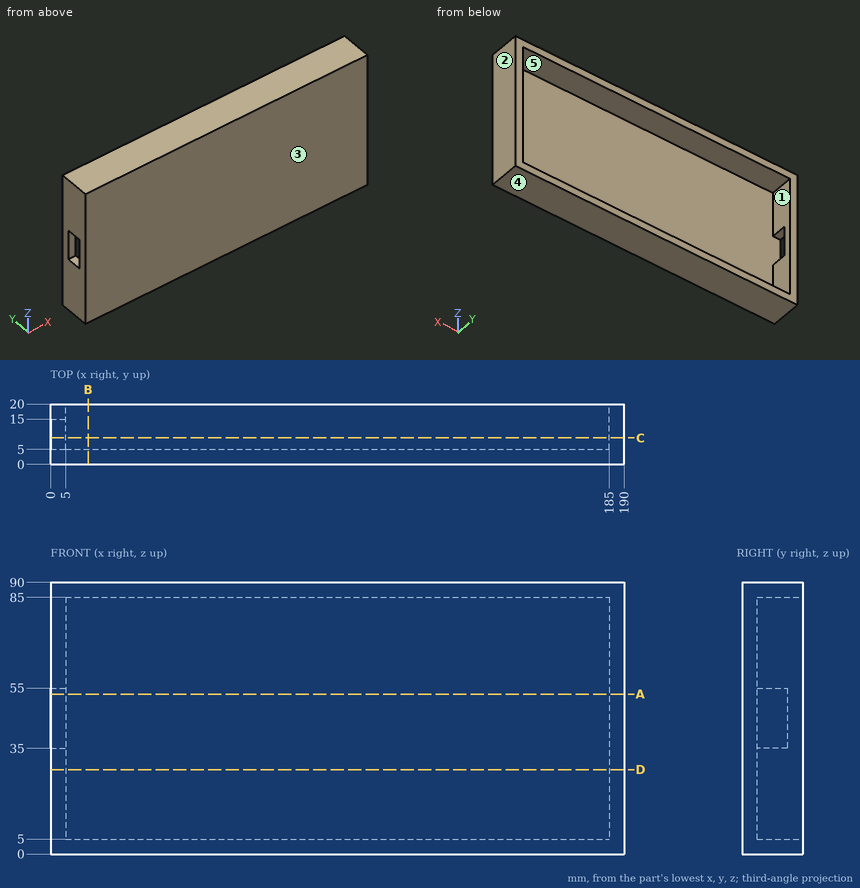
Verification items for this drawing (mm, ordinates from the low corner). A direction names the side the tool comes from. Coordinates: 2 decimals unless noted, no trailing zeros. Loops run counter-clockwise (first coordinate to the right, second up) from the corner with the lowest first, then second, coordinate; pieces in that order, holes last. Notation, with made-up numbers: (88.25, 82) - (119.25, 82) arc R7 ccw to (119.25, 91) - close; hole circle Ø4 at (17, 87.25). An arc over 180 degrees is marked (long way). Use one line per item in the form item = value. Start each with the question number.
Item 1: Section check D-D, the plane z = 28. Enter the section's corners in (x, y), and give its area (3 significant figures).
Item 2: Gauge pin test, flat ends, axial feed: pin 1 (6 mm diameter, centred on x = 148.5, z = 19, fed in from -Y); pin 2 (6 mm diameter, centred on x = 137.5, z = 73, fed in from +Y); pin 3 (4.5 mm diameter, centred on y = 12, z = 38, fed in from -X). Record the tip position at first contact, or that the pin passes through.
Item 3: Tool access check on the marked faces 4 and 5. Record the directions out of +Z, -Z, +X, -X, +Y, -Y that give a thin tool (end or side, any length) a straight path to the whole face; none if there is none.
Item 4: Section check A-A, the plane z = 53. Enter the section's corners in (x, y).
Item 5: Mould release check, pull along X, two halves, no side actions. Record for the marked faces 1, 2 and 3: +X half, -X half, draft (parallel to the pull), parting line (faces both ways), or undercut.
Item 6: Section check B-B, the plane x = 12.5. Enter the section's corners in (y, z), and give its area (3 significant figures).
Item 7: Section check C-C, the plane y = 8.75. Enter the section's corners in (x, z).
Item 8: Thickness scan on probe 1 along Z at (x, y) = (48.5, 11.75); probe 2 along X at (y, z) = (17.5, 22); probe 3 along Y at (x, z) = (23.5, 62). Record the ranges inside material, lowest first.
Computed:
q1.outline = (0, 0) - (190, 0) - (190, 20) - (185, 20) - (185, 5) - (5, 5) - (5, 20) - (0, 20) - close
q1.area = 1,100 mm2
q2.pin_1 = 0
q2.pin_2 = 5
q2.pin_3 = 185
q3.face_4 = -Z, +X, -X, +Y, -Y
q3.face_5 = +Y
q4.outline = (0, 0) - (190, 0) - (190, 20) - (185, 20) - (185, 5) - (0, 5) - close; (0, 15) - (5, 15) - (5, 20) - (0, 20) - close
q5.face_1 = undercut
q5.face_2 = +X half
q5.face_3 = draft
q6.outline = (0, 0) - (20, 0) - (20, 5) - (5, 5) - (5, 85) - (20, 85) - (20, 90) - (0, 90) - close
q6.area = 600 mm2
q7.outline = (0, 0) - (190, 0) - (190, 90) - (0, 90) - (0, 55) - (5, 55) - (5, 85) - (185, 85) - (185, 5) - (5, 5) - (5, 35) - (0, 35) - close
q8.probe_1 = 0 to 5, 85 to 90
q8.probe_2 = 0 to 5, 185 to 190
q8.probe_3 = 0 to 5
